Here's the drawing with two shaded views (mm, measured from the low corner). I have some questions. A direction names the side the tool comes from. Round coordinates to 2 decimals unless told otherwise and drop trailing zeros. Loops run counter-clockwise (first coordinate to the right, second up) from the corner with the lowest first, then second, coordinate; pieces in that order, holes last.
(1) I want a section at A-A on y = 91. Write out the boundary of the cut face in (x, z), plus the area to 3 significant figures.
(2) If I drill on line 1 along X through (y, z) = (79, 58); line 2 along X through (y, z) = (8, 54) (1 decimal); line 3 along Z through (x, y) = (135, 108.5), over which ranges is the centre line in solid material (lowest first)?
(3) Which directions (+Z, -Z, +X, -X, +Y, -Y) give clear straight access to the entire face, cutting with the end or side of a thin tool? Please do the marked faces 4, 5 and 6.
(4) I want a section at D-D on x = 22. Write out the boundary of the cut face in (y, z), plus the area to 3 significant figures.
(5) I want a section at B-B on x = 101. Write out the boundary of the cut face in (y, z).
(6) I want a section at C-C on y = 27. Write out the boundary of the cut face in (x, z), plus the area to 3 significant figures.
(7) Thinking about a two-plate mould opening in Z: for the marked faces 1, 2 and 3, which applies, released by +Z, released by -Z, zero draft, split by the parting line, or undercut?
(8) Will these pins go through, and if not, where does the flat tip stop? pin 1 Ø13 at (y, z) = (105, 42.5) entering from -X; pin 2 Ø12 at (x, z) = (25.85, 58) entering from +Y; pin 3 Ø11.5 at (x, z) = (32, 53.5) entering from +Y.
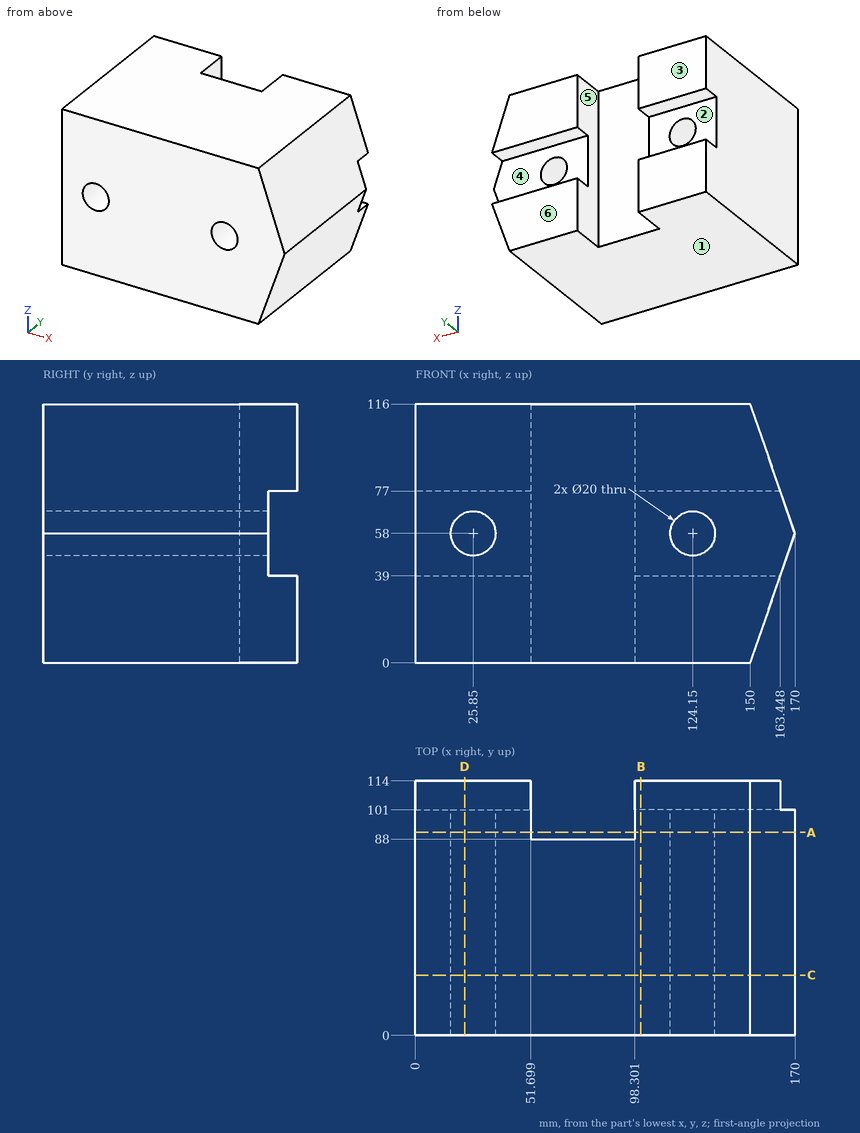
Filled sheet:
1. outline: (0, 0) - (51.7, 0) - (51.7, 116) - (0, 116) - close; (98.3, 0) - (150, 0) - (170, 58) - (150, 116) - (98.3, 116) - close; hole circle Ø20 at (25.85, 58); hole circle Ø20 at (124.15, 58)
1. area: 12,500 mm2
2. line 1: x = 0 to 15.85, 35.85 to 114.15, 134.15 to 170
2. line 2: x = 0 to 16.7, 35 to 115, 133.3 to 168.6
2. line 3: z = 0 to 39, 77 to 116
3. face 4: +X, -X, +Y
3. face 5: +Z, -Z, +Y
3. face 6: +Z, -Z, +X, -X, +Y
4. outline: (0, 0) - (114, 0) - (114, 39) - (101, 39) - (101, 48.77) - (0, 48.77) - close; (0, 67.23) - (101, 67.23) - (101, 77) - (114, 77) - (114, 116) - (0, 116) - close
4. area: 10,900 mm2
5. outline: (0, 0) - (114, 0) - (114, 39) - (101, 39) - (101, 77) - (114, 77) - (114, 116) - (0, 116) - close
6. outline: (0, 0) - (150, 0) - (170, 58) - (150, 116) - (0, 116) - close; hole circle Ø20 at (25.85, 58); hole circle Ø20 at (124.15, 58)
6. area: 17,900 mm2
7. face 1: released by -Z
7. face 2: undercut
7. face 3: zero draft
8. pin 1: stops at x = 0
8. pin 2: passes through
8. pin 3: stops at y = 101
